```python
from build123d import *

# Parameters (mm, degrees)
SKETCH1_R               = 5
BOSS_EXTRUDE1_DEPTH     = 122
SKETCH2_R               = 4
BOSS_EXTRUDE2_DEPTH     = 10
SKETCH3_R               = 2.5
CUT_EXTRUDE1_DEPTH      = 6
CUT_EXTRUDE1_DEPTH_BACK = 6


with BuildPart() as part:
    # Sketch1 → Boss-Extrude1 (new body)
    with BuildSketch(Plane.XY):
        Circle(SKETCH1_R)
    extrude(amount=BOSS_EXTRUDE1_DEPTH)

    # Sketch2 → Boss-Extrude2 (add)
    with BuildSketch(Plane(origin=(0, 0, 0), x_dir=(-1, 0, 0), z_dir=(0, 0, -1))):
        Circle(SKETCH2_R)
    extrude(amount=BOSS_EXTRUDE2_DEPTH)

    # Sketch3 → Cut-Extrude1 (cut, two sides)
    with BuildSketch(Plane(origin=(0, 0, 0), x_dir=(0, 0, -1), z_dir=(1, 0, 0))) as cut_extrude1_sk:
        with Locations((5, 0)):
            Circle(SKETCH3_R)
    extrude(amount=CUT_EXTRUDE1_DEPTH, mode=Mode.SUBTRACT)
    extrude(cut_extrude1_sk.sketch, amount=-CUT_EXTRUDE1_DEPTH_BACK, mode=Mode.SUBTRACT)


solid = part.part
```
Work out the finished part from the listing and answer in its coordinate system (mm). A direction names the side the tool comes from. Give positions to 0.01 mm unless a question says otherwise; leave off trailing zeros. Order: outer loops, then holes, each group sorted by start corner. A loop starts at its lowest first (then second) coordinate and runs counter-clockwise, first axis right, second up. Notation, with made-up numbers: (-29.5, 4.25) - (-2.5, 4.25) arc R22 cw to (-2.5, 16.25) - close; hole circle Ø8 at (-8, 72). An arc over 180 degrees is marked (long way). One line per item, written item: value. Start each with the question number.
1. Section A-A, the plane y = 0 is taken. Write down the section's boundary in (x, z), then the cut area to 3 significant figures.
2. Which of the six approach directions +Z, -Z, +X, -X, +Y, -Y give full straight-line access (tool end or side, diameter ignored) to faces 1 (the face through (0, 0, 122)), 2 (the face through (2.95, 2.7, -4.93))?
3. Consider line 1 (Z direction, x = 0.5, y = 0); line 2 (Y direction, x = 0.25, z = -5); line 3 (Y direction, x = -1.75, z = -5). Determine where each line is inside the solid, lowest interval first.
4. Section D-D, the plane z = 59 is taken. Write down the section's boundary in (x, y).
5. Section B-B, the plane x = 0 is taken. Write down the section's boundary in (y, z), then the cut area to 3 significant figures.
6. Section C-C, the plane z = -5 is taken. Write down the section's boundary in (x, y).
7. Each of these flat-tipped pins is pushed along its axis until it touches: pin 1 Ø4.5 at (y, z) = (0, -5) entering from -X; pin 2 Ø4 at (x, z) = (3.5, 86.5) entering from +Y; pin 3 Ø3 at (x, z) = (-3, 20.5) entering from -Y; pin 4 Ø3 at (x, y) = (4, 3.5) entering from +Z. Where does it stop, or does it pass through?
Filled sheet:
1. outline: (-5, 0) - (-4, 0) - (-4, -2.5) - (4, -2.5) - (4, 0) - (5, 0) - (5, 122) - (-5, 122) - close; (-4, -10) - (4, -10) - (4, -7.5) - (-4, -7.5) - close
1. area: 1,260 mm²
2. face 1: +Z, +X, -X, +Y, -Y
2. face 2: -Z
3. line 1: -10 to -7.5, -2.5 to 122
3. line 2: -3.99 to -2.5, 2.5 to 3.99
3. line 3: -3.6 to -2.5, 2.5 to 3.6
4. outline: circle Ø10 at (0, 0)
5. outline: (-5, 0) - (-4, 0) - (-4, -10) - (4, -10) - (4, 0) - (5, 0) - (5, 122) - (-5, 122) - close; hole circle Ø5 at (0, -5)
5. area: 1,280 mm²
6. outline: (-3.12, -2.5) arc R4 ccw to (3.12, -2.5) - close; (-3.12, 2.5) - (3.12, 2.5) arc R4 ccw to start
7. pin 1: through
7. pin 2: y = 4.77
7. pin 3: y = -4.77
7. pin 4: z = 122
